Here's the drawing with two shaded views (mm, measured from the low corner). I have some questions. Coordinates: 2 decimals unless noted, no trailing zeros. Order: outer loops, then holes, each group sorted by start corner. A loop starts at its lowest first (then second) coordinate and runs counter-clockwise, first axis right, second up. Notation, with made-up numbers: (6, 53.25) -> (46, 53.25) arc R8 cw to (46, 66.25) -> close; hole circle Ø11 at (7, 37). An arc over 180 degrees is marked (long way). One line per item, written item: value. Start each with the question number.
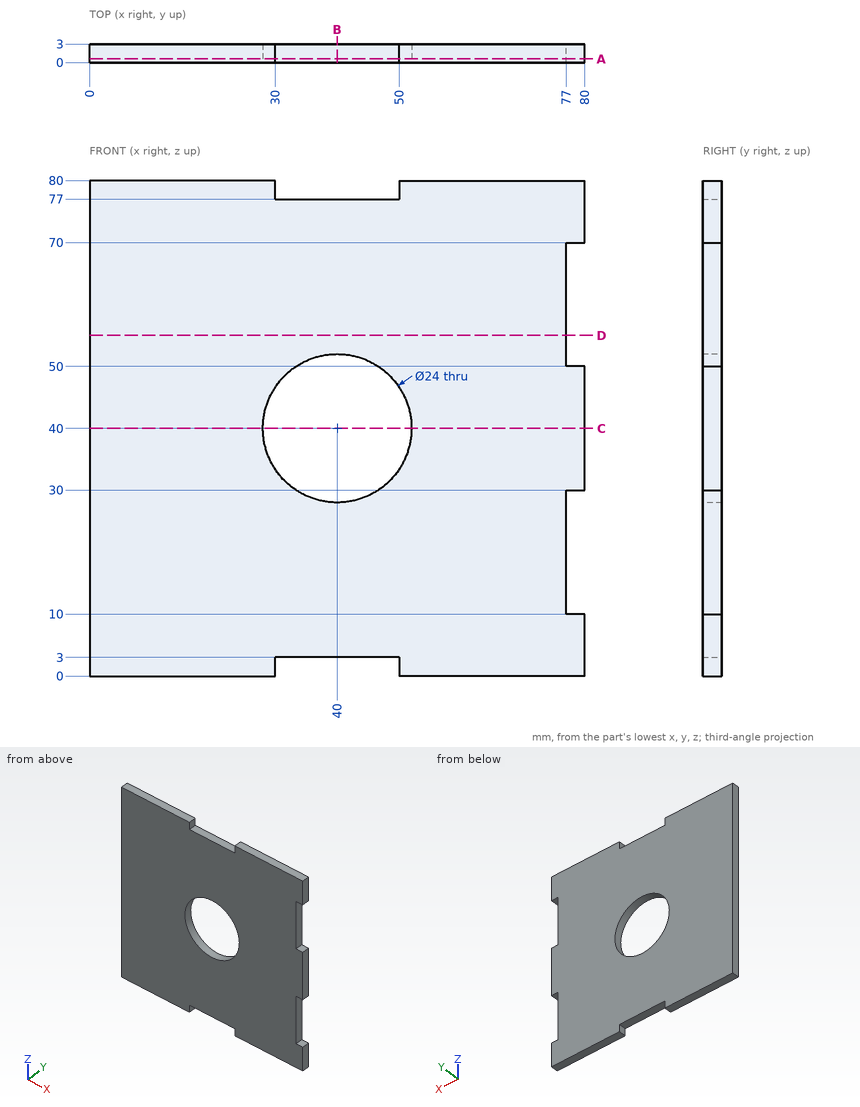
Q1. Imagine slicing it at A-A (y = 0.6). Write out the boundary of the cut face in (x, z).
Q2. For P1, Ø1.5, axis at x = 40.5, y = 1.5, coming from the -Z side; P2, Ø0.9, axis at y = 2, z = 22, coming from the +X side, each with a flat end and sliding along its axis, tell me the tip position at first contact or that it passes through.
Q3. Imagine slicing it at C-C (z = 40). Write out the boundary of the cut face in (x, y).
Q4. Imagine slicing it at B-B (x = 40). Write out the boundary of the cut face in (y, z).
Q5. Imagine slicing it at D-D (z = 55). Write out the boundary of the cut face in (x, y).
Q6. I need wall thicknesses on line 1 (X direction, y = 2.05, z = 40); line 2 (X direction, y = 1.1, z = 27); line 3 (Z direction, x = 37, y = 2.4). Which ranges of each line are inside material? Lowest first, please.
Completed:
1. outline: (0, 0) -> (30, 0) -> (30, 3) -> (50, 3) -> (50, 0) -> (80, 0) -> (80, 10) -> (77, 10) -> (77, 30) -> (80, 30) -> (80, 50) -> (77, 50) -> (77, 70) -> (80, 70) -> (80, 80) -> (50, 80) -> (50, 77) -> (30, 77) -> (30, 80) -> (0, 80) -> close; hole circle Ø24 at (40, 40)
2. P1: stops at z = 3
2. P2: stops at x = 77
3. outline: (0, 0) -> (28, 0) -> (28, 3) -> (0, 3) -> close; (52, 0) -> (80, 0) -> (80, 3) -> (52, 3) -> close
4. outline: (0, 3) -> (3, 3) -> (3, 28) -> (0, 28) -> close; (0, 52) -> (3, 52) -> (3, 77) -> (0, 77) -> close
5. outline: (0, 0) -> (77, 0) -> (77, 3) -> (0, 3) -> close
6. line 1: x = 0 to 28, 52 to 80
6. line 2: x = 0 to 77
6. line 3: z = 3 to 28.38, 51.62 to 77
